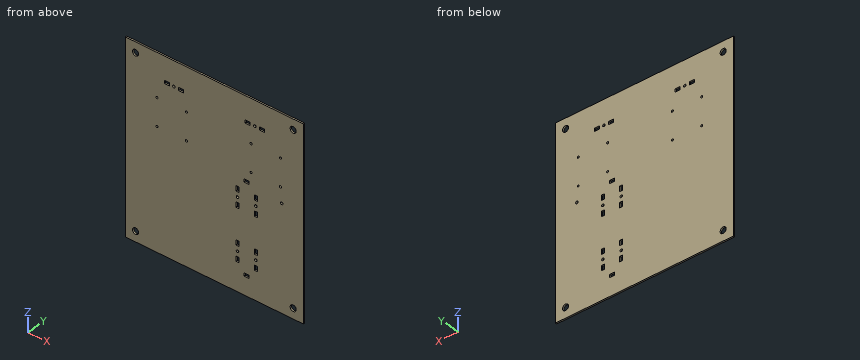
Autodesk Inventor part; units mm, degrees
ref_plane "YZ Plane" through (0, 0, 0) normal (1, 0, 0) x (0, 1, 0)
ref_plane "XZ Plane" through (0, 0, 0) normal (0, 1, 0) x (-1, 0, 0)
ref_plane "XY Plane" through (0, 0, 0) normal (0, 0, 1) x (1, 0, 0)
sketch "Boceto1" plane through (0, 0, 0) normal (0, 1, 0) x (-1, 0, 0)
  line L0 (0, 0) -> (350, 0)
  line L1 (350, 0) -> (350, -370)
  line L2 (350, -370) -> (0, -370)
  line L3 (0, -370) -> (0, 0)
  circle A0 centre (20, -350) radius 6
  circle A1 centre (254.5115, -48) radius 2.5
  circle A2 centre (95.4885, -48) radius 2.5
  line L4 (245.5005, -51) -> (235.5005, -51)
  line L5 (235.5005, -51) -> (235.5005, -45)
  line L6 (235.5005, -45) -> (245.5005, -45)
  line L7 (245.5005, -45) -> (245.5005, -51)
  line L8 (273.5005, -51) -> (263.5005, -51)
  line L9 (263.5005, -51) -> (263.5005, -45)
  line L10 (263.5005, -45) -> (273.5005, -45)
  line L11 (273.5005, -45) -> (273.5005, -51)
  line L12 (114.4775, -51) -> (104.4775, -51)
  line L13 (104.4775, -51) -> (104.4775, -45)
  line L14 (104.4775, -45) -> (114.4775, -45)
  line L15 (114.4775, -45) -> (114.4775, -51)
  line L16 (86.4775, -51) -> (76.4775, -51)
  line L17 (76.4775, -51) -> (76.4775, -45)
  line L18 (76.4775, -45) -> (86.4775, -45)
  line L19 (86.4775, -45) -> (86.4775, -51)
  line L20 (254.5115, -48) -> (95.4885, -48) construction
  line L21 (114.4775, -45) -> (129.4775, -45) construction
  line L22 (129.4775, -45) -> (129.4775, -295) construction
  circle A3 centre (129.4775, -295) radius 2.5
  line L23 (132.4775, -315) -> (126.4775, -315)
  line L24 (126.4775, -315) -> (126.4775, -305)
  line L25 (126.4775, -305) -> (132.4775, -305)
  line L26 (132.4775, -305) -> (132.4775, -315)
  line L27 (132.4775, -285) -> (126.4775, -285)
  line L28 (126.4775, -285) -> (126.4775, -275)
  line L29 (126.4775, -275) -> (132.4775, -275)
  line L30 (132.4775, -275) -> (132.4775, -285)
  line L31 (132.4775, -215) -> (126.4775, -215)
  line L32 (126.4775, -215) -> (126.4775, -205)
  line L33 (126.4775, -205) -> (132.4775, -205)
  line L34 (132.4775, -205) -> (132.4775, -215)
  circle A4 centre (129.4775, -195) radius 2.5
  line L35 (132.4775, -185) -> (126.4775, -185)
  line L36 (126.4775, -185) -> (126.4775, -175)
  line L37 (126.4775, -175) -> (132.4775, -175)
  line L38 (132.4775, -175) -> (132.4775, -185)
  line L39 (96.4775, -315) -> (90.4775, -315)
  line L40 (90.4775, -315) -> (90.4775, -305)
  line L41 (90.4775, -305) -> (96.4775, -305)
  line L42 (96.4775, -305) -> (96.4775, -315)
  circle A5 centre (93.4775, -295) radius 2.5
  line L43 (96.4775, -285) -> (90.4775, -285)
  line L44 (90.4775, -285) -> (90.4775, -275)
  line L45 (90.4775, -275) -> (96.4775, -275)
  line L46 (96.4775, -275) -> (96.4775, -285)
  line L47 (96.4775, -215) -> (90.4775, -215)
  line L48 (90.4775, -215) -> (90.4775, -205)
  line L49 (90.4775, -205) -> (96.4775, -205)
  line L50 (96.4775, -205) -> (96.4775, -215)
  line L51 (96.4775, -185) -> (90.4775, -185)
  line L52 (90.4775, -185) -> (90.4775, -175)
  line L53 (90.4775, -175) -> (96.4775, -175)
  line L54 (96.4775, -175) -> (96.4775, -185)
  circle A6 centre (93.4775, -195) radius 2.5
  line L55 (116.4775, -335) -> (106.4775, -335)
  line L56 (106.4775, -335) -> (106.4775, -329)
  line L57 (106.4775, -329) -> (116.4775, -329)
  line L58 (116.4775, -329) -> (116.4775, -335)
  line L59 (116.4775, -161) -> (106.4775, -161)
  line L60 (106.4775, -161) -> (106.4775, -155)
  line L61 (106.4775, -155) -> (116.4775, -155)
  line L62 (116.4775, -155) -> (116.4775, -161)
  circle A7 centre (330, -350) radius 6
  circle A8 centre (330, -20) radius 6
  circle A9 centre (20, -20) radius 6
  line L63 (106.4775, -140) -> (41.4775, -140) construction
  line L64 (41.4775, -140) -> (41.4775, -80) construction
  line L65 (41.4775, -80) -> (106.4775, -80) construction
  line L66 (106.4775, -80) -> (106.4775, -140) construction
  circle A10 centre (42.4775, -166.3418) radius 2.5
  circle A11 centre (102.7945, -137.079) radius 2
  circle A12 centre (45.0335, -137.079) radius 2
  circle A13 centre (45.0335, -83.683) radius 2
  circle A14 centre (102.7945, -83.683) radius 2
  line L67 (291.4775, -140) -> (226.4775, -140) construction
  line L68 (226.4775, -140) -> (226.4775, -80) construction
  line L69 (226.4775, -80) -> (291.4775, -80) construction
  line L70 (291.4775, -80) -> (291.4775, -140) construction
  circle A15 centre (287.7945, -137.079) radius 2
  circle A16 centre (230.0335, -137.079) radius 2
  circle A17 centre (230.0335, -83.683) radius 2
  circle A18 centre (287.7945, -83.683) radius 2
  point P0 (235.5005, -48)
  point P1 (263.5005, -48)
  point P2 (104.4775, -48)
  point P3 (175, 0)
  point P4 (175, -48)
  point P5 (129.4775, -305)
  point P6 (129.4775, -285)
  point P7 (129.4775, -215)
  point P8 (129.4775, -275)
  point P9 (129.4775, -185)
  point P10 (126.4775, -310)
  point P11 (96.4775, -310)
  point P12 (93.4775, -305)
  point P13 (93.4775, -285)
  point P14 (93.4775, -215)
  point P15 (93.4775, -275)
  point P16 (93.4775, -205)
  point P17 (93.4775, -175)
  dimension "d0" = 350
  dimension "d1" = 370
  dimension "d4" = 12
  dimension "d5" = 20
  dimension "d6" = 20
  dimension "d7" = 5
  dimension "d8" = 5
  dimension "d11" = 10
  dimension "d12" = 6
  dimension "d13" = 10
  dimension "d15" = 18
  dimension "d16" = 6
  dimension "d17" = 9.011
  dimension "d18" = 10
  dimension "d19" = 6
  dimension "d20" = 10
  dimension "d21" = 6
  dimension "d22" = 18
  dimension "d23" = 9.011
  dimension "d26" = 121.023
  dimension "d27" = 45
  dimension "d29" = 15
  dimension "d30" = 250
  dimension "d31" = 5
  dimension "d33" = 10
  dimension "d34" = 6
  dimension "d35" = 10
  dimension "d36" = 20
  dimension "d37" = 10
  dimension "d39" = 10
  dimension "d40" = 60
  dimension "d41" = 6
  dimension "d42" = 5
  dimension "d43" = 10
  dimension "d44" = 6
  dimension "d45" = 10
  dimension "d46" = 20
  dimension "d48" = 10
  dimension "d50" = 42
  dimension "d51" = 6
  dimension "d52" = 6
  dimension "d53" = 5
  dimension "d54" = 6
  dimension "d55" = 10
  dimension "d56" = 5
  dimension "d57" = 20
  dimension "d58" = 10
  dimension "d59" = 6
  dimension "d60" = 10
  dimension "d61" = 10
  dimension "d62" = 6
  dimension "d64" = 16
  dimension "d66" = 10
  dimension "d67" = 6
  dimension "d68" = 16
  dimension "d70" = 20
  dimension "d71" = 20
  dimension "d73" = 20
  dimension "d77" = 20
  dimension "d81" = 65
  dimension "d82" = 60
  dimension "d83" = 5
  dimension "d84" = 11.3418
  dimension "d85" = 48
extrude "Extrusión1" add sketch "Boceto1" along normal blind 3
properties part number "BaseProyecto"
The listing builds one solid part. Answer for the finished solid, in the listing's coordinates (mm). Round coordinates to 2 decimals unless told otherwise and drop trailing zeros. Write each loop counter-clockwise with the first axis right and the second up, starting at its lowest first coordinate (ties: lowest second). Pieces come first, ordered by that corner, then holes. Notation, with made-up numbers: (-7.75, -38.5) - (-2.75, -38.5) arc R22 cw to (-2.75, -26.5) - close; hole circle Ø2 at (64, 38). An arc over 180 degrees is marked (long way). Use a Markdown table: item, result. Add a question column.
1. Consider line 1 (Z direction, x = -330, y = 1); line 2 (X direction, y = 1.5, z = -281.5); line 3 (X direction, y = 0.6, z = -295). Determine where each line is inside the solid, lowest interval first.
2. A flat-ended cylindrical pin translates along its axis: P1, Ø4, axis at x = -129.48, z = -195, coming from the -Y side. Find the tip coordinate at first contact, or state that the pin passes through.
3. The part is cut by section A-A (x = -20). Write down the section's boundary in (y, z), and give its area (3 significant figures).
4. The part is cut by section B-B (z = -350). Write down the section's boundary in (x, y), and give its area (3 significant figures).
Reported:
| question | item | result |
|---|---|---|
| 1 | line 1 | -370 to -356, -344 to -26, -14 to 0 |
| 1 | line 2 | -350 to -132.48, -126.48 to -96.48, -90.48 to 0 |
| 1 | line 3 | -350 to -131.98, -126.98 to -95.98, -90.98 to 0 |
| 2 | P1 | through |
| 3 | outline | (0, -370) - (3, -370) - (3, -356) - (0, -356) - close; (0, -344) - (3, -344) - (3, -26) - (0, -26) - close; (0, -14) - (3, -14) - (3, 0) - (0, 0) - close |
| 3 | area | 1,040 mm^2 |
| 4 | outline | (-350, 0) - (-336, 0) - (-336, 3) - (-350, 3) - close; (-324, 0) - (-26, 0) - (-26, 3) - (-324, 3) - close; (-14, 0) - (0, 0) - (0, 3) - (-14, 3) - close |
| 4 | area | 978 mm^2 |
